from build123d import *

# Parameters (mm, degrees)
BOSS_EXTRUDE2_DEPTH = 8
SKETCH2_R           = 6
CUT_EXTRUDE1_DEPTH  = 10


with BuildPart() as part:
    # Sketch1 → Boss-Extrude2 (new body)
    with BuildSketch(Plane(origin=(0, 0, 0), x_dir=(1, 0, 0), z_dir=(0, 1, 0))):
        with BuildLine():
            ThreePointArc((28.779527534, 0), (32.991059726, 5.817213952), (27.043909653, 9.843178132))
            ThreePointArc((27.043909653, 9.843178132), (20.752040899, 11.158464676), (20.954773741, 17.583142917))
            ThreePointArc((20.954773741, 17.583142917), (21.533384924, 25.662488844), (13.677257194, 23.689704368))
            ThreePointArc((13.677257194, 23.689704368), (7.385388439, 22.374417824), (4.99751251, 28.342301843))
            ThreePointArc((4.99751251, 28.342301843), (0, 33.5), (-4.99751251, 28.342301843))
            ThreePointArc((-4.99751251, 28.342301843), (-8.037473368, 22.082776588), (-14.389763767, 24.923801953))
            ThreePointArc((-14.389763767, 24.923801953), (-21.533384924, 25.662488844), (-22.046397143, 18.499123711))
            ThreePointArc((-22.046397143, 18.499123711), (-20.351596989, 11.75), (-27.043909653, 9.843178132))
            ThreePointArc((-27.043909653, 9.843178132), (-32.991059726, 5.817213952), (-28.779527534, 0))
            ThreePointArc((-28.779527534, 0), (-23.316959386, -3.387910912), (-25.704835315, -9.355794932))
            ThreePointArc((-25.704835315, -9.355794932), (-29.011851027, -16.75), (-20.954773741, -17.583142917))
            ThreePointArc((-20.954773741, -17.583142917), (-14.592496609, -18.499123711), (-14.389763767, -24.923801953))
            ThreePointArc((-14.389763767, -24.923801953), (-11.457674801, -31.479702796), (-4.99751251, -28.342301843))
            ThreePointArc((-4.99751251, -28.342301843), (0, -23.5), (4.99751251, -28.342301843))
            ThreePointArc((4.99751251, -28.342301843), (11.457674801, -31.479702796), (14.389763767, -24.923801953))
            ThreePointArc((14.389763767, -24.923801953), (15.105508828, -18.002044413), (22.046397143, -18.499123711))
            ThreePointArc((22.046397143, -18.499123711), (29.011851027, -16.75), (27.043909653, -9.843178132))
            ThreePointArc((27.043909653, -9.843178132), (23.142982196, -4.080732175), (28.779527534, 0))
        make_face()
    extrude(amount=BOSS_EXTRUDE2_DEPTH)

    # Sketch2 → Cut-Extrude1 (cut)
    with BuildSketch(Plane(origin=(0, 8, 0), x_dir=(1, 0, 0), z_dir=(0, 1, 0))):
        Circle(SKETCH2_R)
    extrude(amount=-CUT_EXTRUDE1_DEPTH, mode=Mode.SUBTRACT)


solid = part.part
Can you work these out from the model? Positions are in its coordinate system, mm. Coordinates: 2 decimals unless noted, no trailing zeros. Write each loop counter-clockwise with the first axis right and the second up, starting at its lowest first coordinate (ties: lowest second). Pieces come first, ordered by that corner, then holes. Notation, with made-up numbers: (-27.75, 45.25) -> (31.25, 45.25) arc R19 cw to (31.25, 52.25) -> close; hole circle Ø2 at (77.25, -19.5). An arc over 180 degrees is marked (long way). Write each question's results on one line, items separated by ' | '. Start each with the question number.
Q1. If I drill on probe 1 along Z at (x, y) = (0, 4.25); probe 2 along X at (y, z) = (5, 29.5); probe 3 along X at (y, z) = (4.5, 18), over which ranges is the centre line in solid material (lowest first)?
Q2. Imagine slicing it at A-A (x = 0). Write out the boundary of the cut face in (y, z).
Q3. Imagine slicing it at B-B (y = 5.25). Write out the boundary of the cut face in (x, z), then the cut area to 3 significant figures.
Q4. Imagine slicing it at D-D (z = -14.25). Write out the boundary of the cut face in (x, y), then the cut area to 3 significant figures.
Q5. We'd pull the mould along X, two halves only. Please class faces 1 (the face through (-0.1, 3.9, 23.5)), 2 (the face through (0.1, 3.9, -33.5)), 3 (the face through (7, 8, -1)): +X half, -X half, draft (parallel to the pull), parting line (faces both ways), or undercut.
Q6. I'm going to push flat-ended pins straight in: pin 1 (1.5 mm diameter, centred on y = 5.5, z = 6.5, fed in from +X); pin 2 (1 mm diameter, centred on y = 3, z = -22.5, fed in from +X); pin 3 (1.5 mm diameter, centred on y = 4, z = 16.5, fed in from +X); pin 4 (6 mm diameter, centred on x = 23.5, z = 25, fed in from -Y). Where does each tip first touch, or does it pass through?
Q7. Imagine slicing it at C-C (z = 1). Write out the boundary of the cut face in (x, y).
Taken from the geometry:
1) probe 1: z = -33.5 to -6, 6 to 23.5 | probe 2: x = -13.94 to -5.55, 5.55 to 13.94 | probe 3: x = -27.99 to -21.37, -15.11 to 15.11, 21.53 to 27.99
2) outline: (0, -33.5) -> (8, -33.5) -> (8, -6) -> (0, -6) -> close; (0, 6) -> (8, 6) -> (8, 23.5) -> (0, 23.5) -> close
3) outline: (-28.78, 0) arc R5 ccw (long way) to (-27.04, -9.84) arc R5 cw to (-22.05, -18.5) arc R5 ccw (long way) to (-14.39, -24.92) arc R5 cw to (-5, -28.34) arc R5 ccw (long way) to (5, -28.34) arc R5 cw to (13.68, -23.69) arc R5 ccw (long way) to (20.95, -17.58) arc R5 cw to (27.04, -9.84) arc R5 ccw (long way) to (28.78, 0) arc R5 cw to (27.04, 9.84) arc R5 ccw (long way) to (22.05, 18.5) arc R5 cw to (14.39, 24.92) arc R5 ccw (long way) to (5, 28.34) arc R5 cw to (-5, 28.34) arc R5 ccw (long way) to (-14.39, 24.92) arc R5 cw to (-20.95, 17.58) arc R5 ccw (long way) to (-25.7, 9.36) arc R5 cw to start; hole circle Ø12 at (0, 0) | area: 2,470 mm^2
4) outline: (-19.68, 0) -> (19.68, 0) -> (19.68, 8) -> (-19.68, 8) -> close | area: 315 mm^2
5) face 1: undercut | face 2: parting line | face 3: draft
6) pin 1: stops at x = 23.63 | pin 2: stops at x = 23.32 | pin 3: stops at x = 29.45 | pin 4: passes through
7) outline: (-25, 0) -> (-5.92, 0) -> (-5.92, 8) -> (-25, 8) -> close; (5.92, 0) -> (25, 0) -> (25, 8) -> (5.92, 8) -> close
